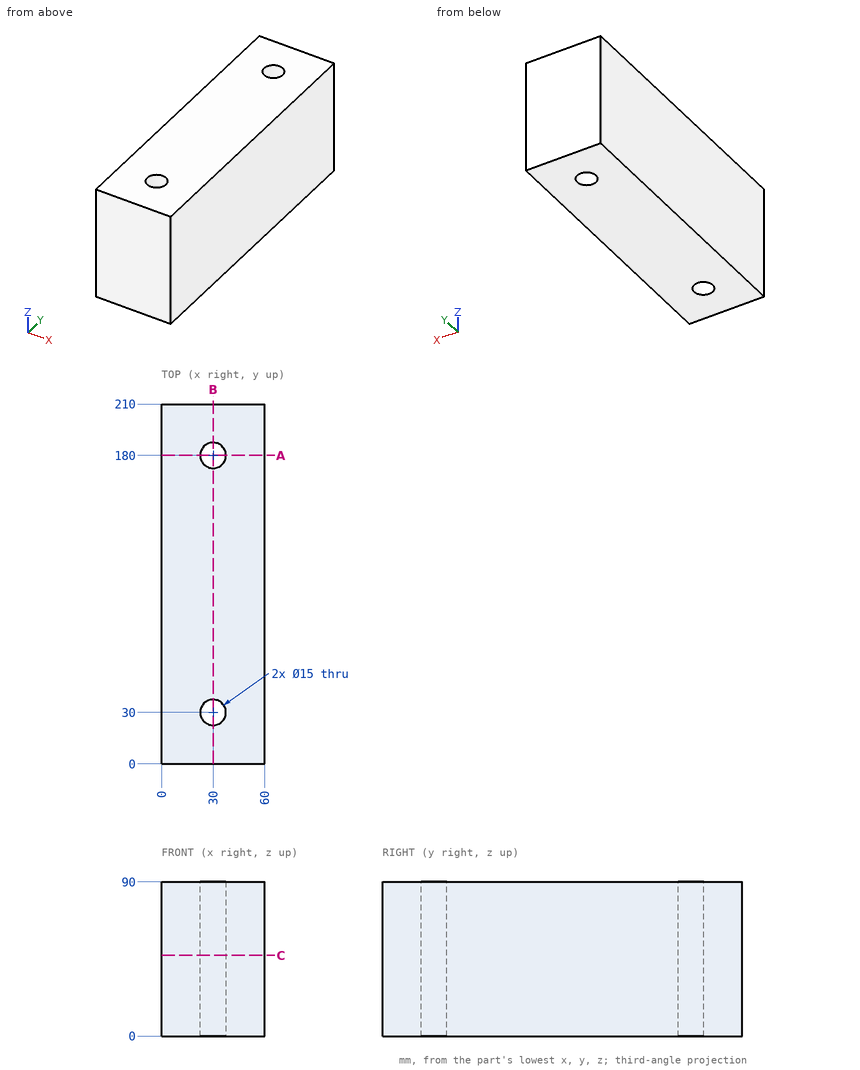
Geometry check sheet. Reference: drawing and pictorial views, mm from the part's lowest x, y, z. Give positions to 0.01 mm unless a question says otherwise; leave off trailing zeros. Order: outer loops, then holes, each group sorted by start corner. A loop starts at its lowest first (then second) coordinate and runs counter-clockwise, first axis right, second up. Notation, with made-up numbers: M -38.75,60.25 L 9.25,60.25 A29 cw 9.25,97.25 Z; hole C 6.5,38.5 d3. An arc over 180 degrees is marked long. Answer in a Markdown table with one row per item. Add a question column.
Item 1: Section check B-B, the plane x = 30. Enter the section's corners in (y, z).
Item 2: Scan lines: probe 1 along Y at (x, z) = (30, 66); probe 2 along Y at (x, z) = (25, 79.5); probe 3 along X at (y, z) = (24, 65.5). Record each from-to range of solid material in increasing order. Write a range as from..to.
Item 3: Gauge pin test, flat end, axial feed: pin 1 (9 mm diameter, centred on x = 30, y = 180, fed in from +Z). Record the tip position at first contact, or that the pin passes through.
Item 4: Section check A-A, the plane y = 180. Enter the section's corners in (x, z).
Item 5: Section check C-C, the plane z = 47. Enter the section's corners in (x, y).
Filled sheet:
| question | item | result |
|---|---|---|
| 1 | outline | M 0,0 L 22.5,0 L 22.5,90 L 0,90 Z; M 37.5,0 L 172.5,0 L 172.5,90 L 37.5,90 Z; M 187.5,0 L 210,0 L 210,90 L 187.5,90 Z |
| 2 | probe 1 | y = 0..22.5, 37.5..172.5, 187.5..210 |
| 2 | probe 2 | y = 0..24.41, 35.59..174.41, 185.59..210 |
| 2 | probe 3 | x = 0..25.5, 34.5..60 |
| 3 | pin 1 | passes through |
| 4 | outline | M 0,0 L 22.5,0 L 22.5,90 L 0,90 Z; M 37.5,0 L 60,0 L 60,90 L 37.5,90 Z |
| 5 | outline | M 0,0 L 60,0 L 60,210 L 0,210 Z; hole C 30,30 d15; hole C 30,180 d15 |
